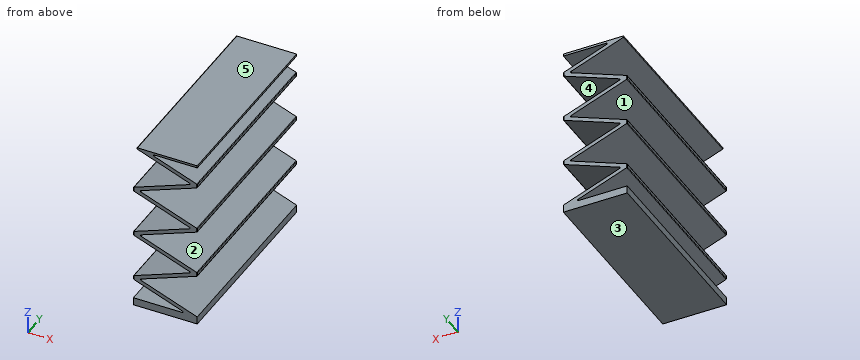
```python
from build123d import *

# Parameters (mm, degrees)
F1_DEPTH = 25
F2_R     = 0.2
F3_R     = 0.2


with BuildPart() as f1:
    # F0 (on Front) → F1 (new body, symmetric)
    with BuildSketch(Plane.XZ):
        Polygon((-8.317317, 2), (-8.317317, 0), (8.317317, 0), (8.317317, 2), (5.515711, 2), align=None)
        Polygon((-8.317317, 7.285714), (5.515711, 2), (8.317317, 2), (-6.82424, 7.785714), (8.317317, 13.571429), (8.317317, 14.571429), (-6.82424, 20.357143), (8.317317, 26.142857), (8.317317, 27.142857), (-6.82424, 32.928571), (8.317317, 38.714286), (8.317317, 39.714286), (-3.974019, 44.410907), (8.317317, 44.410907), (8.317317, 45), (-8.317317, 45), (6.82424, 39.214286), (-8.317317, 33.428571), (-8.317317, 32.428571), (6.82424, 26.642857), (-8.317317, 20.857143), (-8.317317, 19.857143), (6.82424, 14.071429), (-8.317317, 8.285714), align=None)
    extrude(amount=F1_DEPTH, both=True)

    # F2
    f2_edges = [f1.edges().sort_by_distance(p)[0] for p in [
        (-6.82424, 0, 32.928571),
        (-3.974019, 0, 44.410907),
        (-6.82424, 0, 20.357143),
        (-6.82424, 0, 7.785714),
        (5.515711, 0, 2),
        (6.82424, 0, 14.071429),
        (6.82424, 0, 26.642857),
        (6.82424, 0, 39.214286),
    ]]
    fillet(f2_edges, radius=F2_R)

    # F3
    f3_edges = [f1.edges().sort_by_distance(p)[0] for p in [
        (-8.317317, 0, 8.285714),
        (-8.317317, 25, 7.785714),
        (-8.317317, 0, 7.285714),
        (-8.317317, -25, 7.785714),
        (-8.317317, 0, 20.857143),
        (-8.317317, 25, 20.357143),
        (-8.317317, 0, 19.857143),
        (-8.317317, -25, 20.357143),
        (-8.317317, 25, 32.928571),
        (-8.317317, 0, 32.428571),
        (-8.317317, -25, 32.928571),
        (-8.317317, 0, 33.428571),
        (-8.317317, 0, 45),
        (8.317317, 0, 38.714286),
        (8.317317, 25, 39.214286),
        (8.317317, 0, 39.714286),
        (8.317317, -25, 39.214286),
        (8.317317, 0, 26.142857),
        (8.317317, 25, 26.642857),
        (8.317317, 0, 27.142857),
        (8.317317, -25, 26.642857),
        (8.317317, 0, 13.571429),
        (8.317317, 25, 14.071429),
        (8.317317, 0, 14.571429),
        (8.317317, -25, 14.071429),
    ]]
    fillet(f3_edges, radius=F3_R)


solid = f1.part
```
Part model, mm, in its own coordinate system. Face numbers are marked on the shaded views. A direction names the side the tool comes from. Give positions to 0.01 mm unless a question says otherwise; leave off trailing zeros. Order: outer loops, then holes, each group sorted by start corner. A loop starts at its lowest first (then second) coordinate and runs counter-clockwise, first axis right, second up. Notation, with made-up numbers: M -10.75,70.25 L 5.25,70.25 A18 ccw 5.25,98.25 Z; hole C 84.25,-31.5 d6. An arc over 180 degrees is marked long. Use a Markdown table: item, result. Add a question column.
(1) Saw through at A-A, the plane x = 1. Give the number of separate pieces and of enclosed holes in the cut face, and give its area (3 significant figures).
(2) Drop a flat-ended pin along its axis: P1, Ø5, axis at x = -5.5, z = 13, coming from the +Y side. Give the stop position or say it passes through.
(3) 3-axis set-ups, long thin cutter, end or side, ignore diameter. For the marked faces 1 and 2: which of +Z, -Z, +X, -X, +Y, -Y reach the whole face in a straight line?
(4) Probe line 1 along Z through (x, y) = (-7, 23); line 2 along Z through (x, y) = (6.5, -10.5); line 3 along X through (y, z) = (-20, 33). List the from-to ranges inside material, lowest first. Write a range as [from, to].
(5) Mould opens along Z. For the marked faces 3, 4 and 5 say: +Z half, -Z half, draft (parallel to the pull), parting line (faces both ways), or undercut.
(6) Saw through at B-B, the plane z = 35. Give the cut face in (x, y).
Answer key:
| question | item | result |
|---|---|---|
| 1 | separate pieces | 9 |
| 1 | enclosed holes | 0 |
| 1 | area | 504 mm^2 |
| 2 | P1 | through |
| 3 | face 1 | -X, +Y, -Y |
| 3 | face 2 | +X, +Y, -Y |
| 4 | line 1 | [0, 2], [6.78, 8.79], [19.35, 21.36], [31.93, 33.93], [44.5, 45] |
| 4 | line 2 | [0, 2.69], [12.88, 15.27], [25.45, 27.84], [38.02, 40.41], [44.41, 45] |
| 4 | line 3 | [-8.32, -6.45] |
| 5 | face 3 | -Z half |
| 5 | face 4 | undercut |
| 5 | face 5 | +Z half |
| 6 | outline | M -4.2,-25 L -1.4,-25 L -1.4,25 L -4.2,25 Z |
